Source: CAD feature listing. Evaluate the final solid. Frame: model axes, mm. A direction names the side the tool comes from. Round coordinates to 2 decimals unless told otherwise and drop trailing zeros. Write each loop counter-clockwise with the first axis right and the second up, starting at its lowest first coordinate (ties: lowest second). Pieces come first, ordered by that corner, then holes. Notation, with made-up numbers: M 2.25,20.5 L 43.25,20.5 A18 cw 43.25,53.5 Z; hole C -13.75,39 d2. An arc over 180 degrees is marked long. Use a Markdown table: item, result.
```python
from build123d import *

# Parameters (mm, degrees)
BOSS_EXTRUDE3_DEPTH = 7.5
SHELL1_T            = -2.16


with BuildPart() as part:
    # Sketch1 → Boss-Extrude3 (new body)
    with BuildSketch(Plane(origin=(0, 0, 0), x_dir=(1, 0, 0), z_dir=(0, 1, 0))):
        with BuildLine():
            Line((6.867789963, 15.262601487), (8.997617328, -3.918067904))
            ThreePointArc((8.997617328, -3.918067904), (9.024143463, -5.662644076), (8.71939564, -7.380601705))
            Line((8.71939564, -7.380601705), (6.682914815, -14.711932678))
            ThreePointArc((6.682914815, -14.711932678), (5.729593637, -16.117704054), (4.119957175, -16.66))
            Line((4.119957175, -16.66), (-4.119957175, -16.66))
            ThreePointArc((-4.119957175, -16.66), (-5.729593637, -16.117704054), (-6.682914815, -14.711932678))
            Line((-6.682914815, -14.711932678), (-8.71939564, -7.380601705))
            ThreePointArc((-8.71939564, -7.380601705), (-9.024143463, -5.662644076), (-8.997617328, -3.918067904))
            Line((-8.997617328, -3.918067904), (-6.867789963, 15.262601487))
            ThreePointArc((-6.867789963, 15.262601487), (0, 21.41), (6.867789963, 15.262601487))
        make_face()
    extrude(amount=BOSS_EXTRUDE3_DEPTH)

    # Shell1
    shell1_openings = [part.faces().sort_by_distance(p)[0] for p in [
        (0, 7.5, -1.411749104),
    ]]
    offset(amount=SHELL1_T, openings=shell1_openings, kind=Kind.INTERSECTION)


solid = part.part
```
Q1. Section A-A on y = 3. Return loops of the section in (x, z).
Results are:
| item | result |
|---|---|
| outline | M -9,3.92 L -6.87,-15.26 A6.91 ccw 6.87,-15.26 L 9,3.92 A9.16 ccw 8.72,7.38 L 6.68,14.71 A2.66 ccw 4.12,16.66 L -4.12,16.66 A2.66 ccw -6.68,14.71 L -8.72,7.38 A9.16 ccw Z; hole M -6.85,4.16 L -4.72,-15.02 A4.75 ccw 4.72,-15.02 L 6.85,4.16 A7 ccw 6.64,6.8 L 4.6,14.13 A0.5 ccw 4.12,14.5 L -4.12,14.5 A0.5 ccw -4.6,14.13 L -6.64,6.8 A7 ccw Z |
Q2. Section B-B on y = 1. Return loops of the section in (x, z).
Results are:
| item | result |
|---|---|
| outline | M -9,3.92 L -6.87,-15.26 A6.91 ccw 6.87,-15.26 L 9,3.92 A9.16 ccw 8.72,7.38 L 6.68,14.71 A2.66 ccw 4.12,16.66 L -4.12,16.66 A2.66 ccw -6.68,14.71 L -8.72,7.38 A9.16 ccw Z |
Q3. First-contact query: pin 1 Ø1 at (y, z) = (3.5, -6) entering from +X; pin 2 Ø2 at (x, y) = (7, 2) entering from +Z; pin 3 Ø2 at (y, z) = (1.5, -11.5) entering from -X. Flat tips, straight axial feed; report the tip coordinate or a pass-through.
Results are:
| item | result |
|---|---|
| pin 1 | x = 7.95 |
| pin 2 | z = 15.88 |
| pin 3 | x = -7.4 |
Q4. Reachability of faces 4 (the flat face through (0, 5, 14.5)), 5 (the cylindrical face through (-0.14, 3.7, -21.41)) from +Z, -Z, +X, -X, +Y, -Y: full face, straight path, thin tool, end or side. Return the list, or none.
Results are:
| item | result |
|---|---|
| face 4 | +Y |
| face 5 | -Z, +Y, -Y |
Q5. Section C-C on x = 6. Return loops of the section in (y, z).
Results are:
| item | result |
|---|---|
| outline | M 0,-17.93 L 7.5,-17.93 L 7.5,-3.51 L 2.16,-3.51 L 2.16,9.1 L 7.5,9.1 L 7.5,15.88 L 0,15.88 Z |
Q6. Line query: L1, parallel to Z at x = 0.25, y = 3.5; L2, parallel to X at y = 5, z = -15; L3, parallel to X at y = 2.25, z = 5. Output: solid intervals per line, ascending.
Results are:
| item | result |
|---|---|
| L1 | -21.41 to -19.24, 14.5 to 16.66 |
| L2 | -6.9 to -4.72, 4.72 to 6.9 |
| L3 | -9.05 to -6.89, 6.89 to 9.05 |
Q7. Mould query, pull axis X, two halves, no side actions, for faces 1 (the flat face through (-6, 7.5, -5)), 2 (the cylindrical face through (-5.71, 3.7, 16.13)), 3 (the cylindrical face through (-6.87, 4.79, 5.51)). Classes: +X half, -X half, draft (parallel to the pull), parting line (faces both ways), or undercut.
Results are:
| item | result |
|---|---|
| face 1 | draft |
| face 2 | -X half |
| face 3 | undercut |
Q8. Section D-D on z = -1. Return loops of the section in (x, y).
Results are:
| item | result |
|---|---|
| outline | M -8.45,0 L 8.45,0 L 8.45,7.5 L 6.28,7.5 L 6.28,2.16 L -6.28,2.16 L -6.28,7.5 L -8.45,7.5 Z |
